Could you check a few things on this model? Use its own coordinates, in mm. A direction names the side the tool comes from. Give positions to 0.01 mm unless a question says otherwise; leave off trailing zeros. Loops run counter-clockwise (first coordinate to the right, second up) from the corner with the lowest first, then second, coordinate; pieces in that order, holes last. Notation, with made-up numbers: (-32.75, -21.5) - (23.25, -21.5) arc R16 ccw to (23.25, 3.5) - close; hole circle Ø11 at (66, 21). An arc over 180 degrees is marked (long way). Use CSV: the item, a comma, the result in double quotes.
from build123d import *

# Parameters (mm, degrees)
F0_R      = 47.5
F1_DEPTH  = 1.4
F3_W      = 4.9
F3_H      = 4.9
F4_DEPTH  = 1.6
F5_R      = 2
F5_R_2    = 0.95
F6_DEPTH  = 1.401
F7_W      = 27.5
F7_H      = 17
F8_DEPTH  = 10
F9_W      = 14
F9_H      = 23
F10_DEPTH = 3
F11_W     = 8
F11_H     = 8
F12_DEPTH = 2
F13_W     = 6.5
F13_H     = 6.5
F14_DEPTH = 4
F15_R     = 1.932213
F16_DEPTH = 3


with BuildPart() as f1:
    # F0 (on Top) → F1 (new body)
    with BuildSketch(Plane.XY):
        Circle(F0_R)
    extrude(amount=F1_DEPTH)

    # F3 (on face) → F4 (join)
    with BuildSketch(Plane.XY.offset(1.4)):
        with Locations((0, 44.5)):
            Rectangle(F3_W, F3_H)
        Polygon((-22.734278, 35.459238), (-25.614426, 39.423422), (-29.578609, 36.543274), (-26.698461, 32.579091), align=None)
        Polygon((-39.234835, 15.324253), (-43.895012, 16.838436), (-45.409195, 12.178259), (-40.749018, 10.664076), align=None)
        Polygon((-40.749018, -10.664076), (-45.409195, -12.178259), (-43.895012, -16.838436), (-39.234835, -15.324253), align=None)
        Polygon((-26.698461, -32.579091), (-29.578609, -36.543274), (-25.614426, -39.423422), (-22.734278, -35.459238), align=None)
        with Locations((0, -44.5)):
            Rectangle(F3_W, F3_H)
        Polygon((22.734278, -35.459238), (25.614426, -39.423422), (29.578609, -36.543274), (26.698461, -32.579091), align=None)
        Polygon((39.234835, -15.324253), (43.895012, -16.838436), (45.409195, -12.178259), (40.749018, -10.664076), align=None)
        Polygon((40.749018, 10.664076), (45.409195, 12.178259), (43.895012, 16.838436), (39.234835, 15.324253), align=None)
        Polygon((26.698461, 32.579091), (29.578609, 36.543274), (25.614426, 39.423422), (22.734278, 35.459238), align=None)
    extrude(amount=F4_DEPTH)

    # F5 (on face) → F6 (cut, through all)
    with BuildSketch(Plane.XY.offset(1.4)):
        with Locations((-39, 0)):
            Circle(F5_R)
        with Locations((19.5, -33.774991)):
            Circle(F5_R)
        with Locations((19.5, 33.774991)):
            Circle(F5_R)
        with Locations((39, 0)):
            Circle(F5_R_2)
        with Locations((-19.5, 33.774991)):
            Circle(F5_R_2)
        with Locations((-19.5, -33.774991)):
            Circle(F5_R_2)
    extrude(amount=-F6_DEPTH, mode=Mode.SUBTRACT)

    # F7 (on face) → F8 (join)
    with BuildSketch(Plane(origin=(0, 0, 0), x_dir=(1, 0, 0), z_dir=(0, 0, -1))):
        with Locations((0, -30.8)):
            Rectangle(F7_W, F7_H)
    extrude(amount=F8_DEPTH)

    # F9 (on face) → F10 (join)
    with BuildSketch(Plane(origin=(0, 0, 0), x_dir=(1, 0, 0), z_dir=(0, 0, -1))):
        with Locations((-25.821303, -15.041643)):
            Rectangle(F9_W, F9_H)
    extrude(amount=F10_DEPTH)

    # F11 (on face) → F12 (join)
    with BuildSketch(Plane(origin=(0, 0, 0), x_dir=(1, 0, 0), z_dir=(0, 0, -1))):
        with Locations((-0.047592, -0.053598)):
            Rectangle(F11_W, F11_H)
    extrude(amount=F12_DEPTH)

    # F13 (on face) → F14 (join)
    with BuildSketch(Plane(origin=(0, 0, 0), x_dir=(1, 0, 0), z_dir=(0, 0, -1))):
        with Locations((33.2, 0.101188)):
            Rectangle(F13_W, F13_H)
    extrude(amount=F14_DEPTH)

    # F15 (on face) → F16 (join)
    with BuildSketch(Plane(origin=(0, 0, -4), x_dir=(1, 0, 0), z_dir=(0, 0, -1))):
        with Locations((33.285893, 0)):
            Circle(F15_R)
    extrude(amount=F16_DEPTH)


solid = f1.part
1) Suppose I cut it at C-C (z = -8.5). Please give me the cut outline in (x, y).
Answer below:
outline,"(-13.75, 22.3) - (13.75, 22.3) - (13.75, 39.3) - (-13.75, 39.3) - close"
2) Which directions (+Z, -Z, +X, -X, +Y, -Y) give clear straight access to the entire face, cutting with the end or side of a thin tool? Please do faces 1 (the flat face through (-26, 3.542, -1)), 2 (the flat face through (24.69, 34.04, 2.19)), 3 (the flat face through (-26, 15, -3)), 4 (the flat face through (0, 39.3, -5)), 5 (the flat face through (-27.624, -37.963, 2.189)).
Answer below:
face 1,"-Z, -X, -Y"
face 2,"+Z"
face 3,"-Z, -X, +Y, -Y"
face 4,"-Z, +X, -X, +Y"
face 5,"+Z, -X, -Y"
3) Suppose I cut it at B-B (y = 6.5). Please give me the cut outline in (x, z), plus the area to 3 significant figures.
Answer below:
outline,"(-47.05, 0) - (-32.82, 0) - (-32.82, -3) - (-18.82, -3) - (-18.82, 0) - (47.05, 0) - (47.05, 1.4) - (-47.05, 1.4) - close"
area,"174 mm2"
4) I'm going to push flat-ended pins straight in: P1, Ø1.2, axis at y = -0.5, z = -2.5, coming from the +X side; P2, Ø1.5, axis at x = 34.5, z = -5.5, coming from the -Y side; P3, Ø3, axis at x = -19.5, y = 33.77, coming from the -Z side; P4, Ø1.5, axis at x = -19.5, y = -33.77, coming from the -Z side. Where does each tip first touch, or does it pass through?
Answer below:
P1,"stops at x = 36.45"
P2,"stops at y = -1.88"
P3,"stops at z = 0"
P4,"passes through"
5) Suppose I cut it at A-A (x = 19.5). Please give me the cut outline in (y, z) (3 decimals).
Answer below:
outline,"(-43.313, 0) - (-35.775, 0) - (-35.775, 1.4) - (-43.313, 1.4) - close; (-31.775, 0) - (31.775, 0) - (31.775, 1.4) - (-31.775, 1.4) - close; (35.775, 0) - (43.313, 0) - (43.313, 1.4) - (35.775, 1.4) - close"
6) We'd pull the mould along X, two halves only. Please class faces 6 (the flat face through (-24.69, -34.04, 2.19)), 7 (the flat face through (42, -14, 3)), 8 (the flat face through (-28.16, 34.59, 2.19)), 9 (the flat face through (24.195, 37.469, 2.189)): +X half, -X half, draft (parallel to the pull), parting line (faces both ways), or undercut.
Answer below:
face 6,"undercut"
face 7,"draft"
face 8,"-X half"
face 9,"undercut"
7) I need wall thicknesses on line 1 along Y through (x, z) = (19.5, 0.75) (3 decimals); line 2 along Y through (x, z) = (-39, 0.4); line 3 along Z through (x, y) = (-10, 3). Which ranges of each line are inside material? Lowest first, please.
Answer below:
line 1,"y = -43.313 to -35.775, -31.775 to 31.775, 35.775 to 43.313"
line 2,"y = -27.12 to -2, 2 to 27.12"
line 3,"z = 0 to 1.4"
